Check sheet for the drawn part. Datum: minimum x, y, z corner. Units: mm. A direction names the side the tool comes from. Round coordinates to 2 decimals unless told otherwise and drop trailing zeros. Order: outer loops, then holes, each group sorted by start corner. A loop starts at its lowest first (then second) coordinate and runs counter-clockwise, first axis right, second up. Notation, with made-up numbers: (69.5, 14.25) -> (105.5, 14.25) arc R10 ccw to (105.5, 27.25) -> close; hole circle Ø2 at (61.5, -7.75). An arc over 180 degrees is marked (long way). Use CSV: the item, a comma, the result in double quotes.
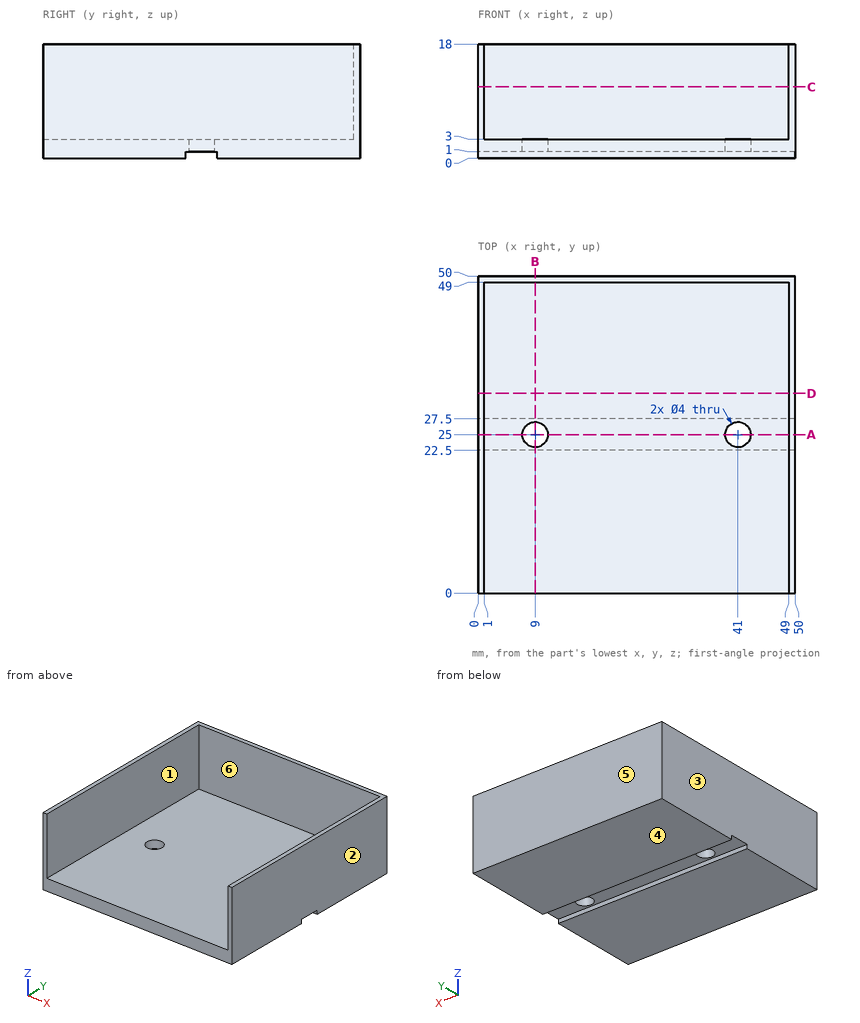
Q1. Sectioned sample at B-B, the plane x = 9. Enter the section's corners in (y, z), then the cut area to 3 significant figures.
Result sheet:
outline,"(0, 0) -> (22.5, 0) -> (22.5, 1) -> (23, 1) -> (23, 3) -> (0, 3) -> close; (27, 1) -> (27.5, 1) -> (27.5, 0) -> (50, 0) -> (50, 18) -> (49, 18) -> (49, 3) -> (27, 3) -> close"
area,"152 mm^2"
Q2. Access from +Z, -Z, +X, -X, +Y, -Y to the whole of each face (thin tool, end or side, straight path). Record for the marked faces 5 and 6.
Result sheet:
face 5,"+Z, -Z, +X, -X, +Y"
face 6,"+Z, -Y"
Q3. Sectioned sample at A-A, the plane y = 25. Enter the section's corners in (x, z).
Result sheet:
outline,"(0, 1) -> (7, 1) -> (7, 3) -> (1, 3) -> (1, 18) -> (0, 18) -> close; (11, 1) -> (39, 1) -> (39, 3) -> (11, 3) -> close; (43, 1) -> (50, 1) -> (50, 18) -> (49, 18) -> (49, 3) -> (43, 3) -> close"
Q4. Sectioned sample at D-D, the plane y = 31.5. Enter the section's corners in (x, z).
Result sheet:
outline,"(0, 0) -> (50, 0) -> (50, 18) -> (49, 18) -> (49, 3) -> (1, 3) -> (1, 18) -> (0, 18) -> close"
Q5. Sectioned sample at C-C, the plane z = 11.25. Enter the section's corners in (x, y), then the cut area to 3 significant figures.
Result sheet:
outline,"(0, 0) -> (1, 0) -> (1, 49) -> (49, 49) -> (49, 0) -> (50, 0) -> (50, 50) -> (0, 50) -> close"
area,"148 mm^2"
Q6. Scan lines: L1, parallel to Y at x = 41, z = 1.5; L2, parallel to X at y = 39, z = 11.25; L3, parallel to Z at x = 32, y = 14. Record each from-to range of solid material in increasing order.
Result sheet:
L1,"y = 0 to 23, 27 to 50"
L2,"x = 0 to 1, 49 to 50"
L3,"z = 0 to 3"
Q7. Go/stop test with flat-tipped pins: pin 1 (6.5 mm diameter, centred on x = 41, y = 25, fed in from -Z); pin 2 (4.5 mm diameter, centred on x = 9, y = 25, fed in from -Z); pin 3 (4 mm diameter, centred on x = 7, z = 14, fed in from -Y); pin 4 (3 mm diameter, centred on x = 24, y = 34, fed in from +Z). Record where each tip stops, or that it passes through.
Result sheet:
pin 1,"stops at z = 0"
pin 2,"stops at z = 1"
pin 3,"stops at y = 49"
pin 4,"stops at z = 3"
Q8. Mould release check, pull along X, two halves, no side actions. Record for the marked faces 1, 2, 3 and 4: pulls with the +X half, pulls with the -X half, needs draft (parallel to the pull), parting line crosses it, or undercut.
Result sheet:
face 1,"undercut"
face 2,"pulls with the +X half"
face 3,"pulls with the -X half"
face 4,"needs draft"
